```python
from build123d import *

# Parameters (mm, degrees)
BASE_EXTRUDE_DEPTH = 12.7
CIRPATTERN1_COUNT  = 2
CIRPATTERN1_ANGLE  = 270


with BuildPart() as part:
    # Sketch1 → Base-Extrude (new, symmetric)
    with BuildSketch(Plane.XY):
        with BuildLine():
            Line((0, 36.5125), (0, 2.6924))
            ThreePointArc((0, 2.6924), (0.788585702, 0.788585702), (2.6924, 0))
            Line((2.6924, 0), (38.5826, 0))
            ThreePointArc((38.5826, 0), (40.486414298, 0.788585702), (41.275, 2.6924))
            Line((41.275, 2.6924), (41.275, 36.5125))
            ThreePointArc((41.275, 36.5125), (36.5125, 41.275), (31.75, 36.5125))
            Line((31.75, 36.5125), (31.75, 35.47745))
            ThreePointArc((31.75, 35.47745), (33.0962, 34.13125), (34.4424, 35.47745))
            Line((34.4424, 35.47745), (34.4424, 36.5125))
            ThreePointArc((34.4424, 36.5125), (36.5125, 38.5826), (38.5826, 36.5125))
            Line((38.5826, 36.5125), (38.5826, 2.6924))
            Line((38.5826, 2.6924), (2.6924, 2.6924))
            Line((2.6924, 2.6924), (2.6924, 36.5125))
            ThreePointArc((2.6924, 36.5125), (4.7625, 38.5826), (6.8326, 36.5125))
            Line((6.8326, 36.5125), (6.8326, 35.47745))
            ThreePointArc((6.8326, 35.47745), (8.1788, 34.13125), (9.525, 35.47745))
            Line((9.525, 35.47745), (9.525, 36.5125))
            ThreePointArc((9.525, 36.5125), (4.7625, 41.275), (0, 36.5125))
        make_face()
    base_extrude = extrude(amount=BASE_EXTRUDE_DEPTH, both=True)

    # CirPattern1: Base-Extrude ×2 about axis
    cirpattern1_axis = Axis((0, 0, 0), (0, 0, 1))
    for i in range(1, CIRPATTERN1_COUNT):
        add(base_extrude.rotate(cirpattern1_axis, i * CIRPATTERN1_ANGLE / (CIRPATTERN1_COUNT - 1)))


solid = part.part
```
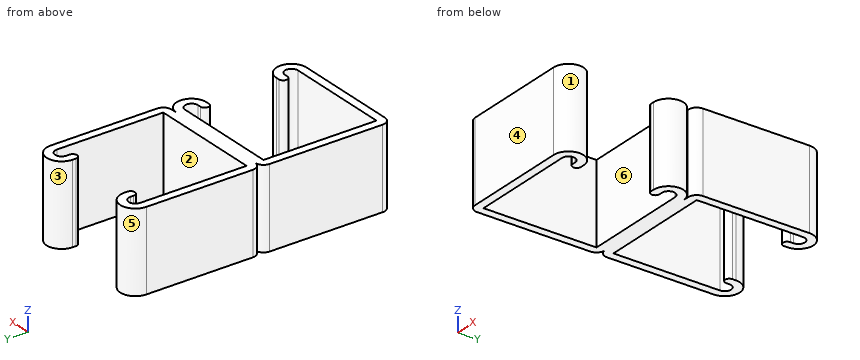
For this review, take the finished solid that the model builds, in its own axes (mm). Face numbers are marked on the shaded views. A direction names the side the tool comes from. Coordinates: 2 decimals unless noted, no trailing zeros. Write each loop counter-clockwise with the first axis right and the second up, starting at its lowest first coordinate (ties: lowest second). Pieces come first, ordered by that corner, then holes. Notation, with made-up numbers: (73.25, 52) -> (99.25, 52) arc R15 ccw to (99.25, 58) -> close; hole circle Ø6 at (-12, -3). An arc over 180 degrees is marked (long way). Put each result on its own line as item: value.
Q1. The part is to be moulded in two halves that separate along Y. For the marked faces 1, 2, 3 and 4, say which applies: +Y half, -Y half, draft (parallel to the pull), parting line (faces both ways), or undercut.
From the geometry:
face 1: undercut
face 2: undercut
face 3: +Y half
face 4: -Y half
Q2. Take a section at A-A, the plane y = 20. State the section outline as (x, z) points (3 decimals), then the cut area to 3 significant figures.
From the geometry:
outline: (0, -12.7) -> (2.692, -12.7) -> (2.692, 12.7) -> (0, 12.7) -> close; (38.583, -12.7) -> (41.275, -12.7) -> (41.275, 12.7) -> (38.583, 12.7) -> close
area: 137 mm2
Q3. Wall thickness on L1, parallel to Y at x = 4.5, z = -10.5 (3 decimals); L2, parallel to X at y = 8, z = 5.25 (3 decimals); L3, parallel to Y at x = 19, z = -4 (3 decimals): over which ranges is each line inside the solid? List them lowest first.
From the geometry:
L1: y = -41.275 to -38.583, -2.692 to 2.692, 38.566 to 41.268
L2: x = 0 to 2.692, 38.583 to 41.275
L3: y = -41.275 to -38.583, -2.692 to 2.692
Q4. Tool access review of the marked faces 5 and 6: name each direction out of +Z, -Z, +X, -X, +Y, -Y from which nothing blocks a thin tool from reaching the whole face with its end or side.
From the geometry:
face 5: +Z, -Z, +Y
face 6: +Z, -Z
Q5. Take a section at C-C, the plane y = -27. State the section outline as (x, z) points, then the cut area to 3 significant figures.
From the geometry:
outline: (0, -12.7) -> (2.69, -12.7) -> (2.69, 12.7) -> (0, 12.7) -> close
area: 68.4 mm2
Q6. Clearance check with flat-ended pins moving along their axes: pin 1 Ø12.5 at (x, z) = (19, -1.5) entering from +Y; pin 2 Ø0.5 at (x, z) = (36, 2.5) entering from +Y; pin 3 Ø7.5 at (y, z) = (-28.5, 3) entering from +X. State where each tip first meets the part, or that it passes through.
From the geometry:
pin 1: stops at y = 2.69
pin 2: stops at y = 41.27
pin 3: stops at x = 38.64
Q7. Take a section at B-B, the plane x = 29. State the section outline as (y, z) points (3 decimals).
From the geometry:
outline: (-41.275, -12.7) -> (-38.583, -12.7) -> (-38.583, 12.7) -> (-41.275, 12.7) -> close; (-2.692, -12.7) -> (2.692, -12.7) -> (2.692, 12.7) -> (-2.692, 12.7) -> close
